Could you check a few things on this model? Use its own coordinates, in mm. Round coordinates to 2 decimals unless told otherwise and drop trailing zeros. Loops run counter-clockwise (first coordinate to the right, second up) from the corner with the lowest first, then second, coordinate; pieces in that order, holes last.
Autodesk Inventor part; units mm, degrees
ref_plane "YZ Plane" through (0, 0, 0) normal (1, 0, 0) x (0, 1, 0)
ref_plane "XZ Plane" through (0, 0, 0) normal (0, 1, 0) x (-1, 0, 0)
ref_plane "XY Plane" through (0, 0, 0) normal (0, 0, 1) x (1, 0, 0)
sketch "Sketch1" plane through (0, 0, 0) normal (0, 1, 0) x (-1, 0, 0)
  line L0 (0, 0) -> (0, -180)
  line L1 (0, -180) -> (-120, -180)
  line L2 (-120, -180) -> (-120, 0)
  line L3 (-120, 0) -> (0, 0)
  dimension "d1" = 180
  dimension "d2" = 120
extrude "Extrusion1" add sketch "Sketch1" along normal blind 1
fillet "Fillet1" radius 2 4 edges at (0, 0.5, 0) (120, 0.5, 0) (120, 0.5, -180) (0, 0.5, -180)
sketch "Sketch2" plane through (0, 1, 0) normal (0, 1, 0) x (1, 0, 0)
  arc A0 (2, 180) -> (0, 178) centre (2, 178) ccw
  circle A1 centre (2.7071, 177.2929) radius 1.5
  line L0 (2, 0) -> (118, 0)
  line L1 (118, 180) -> (2, 180)
  arc A2 (120, 178) -> (118, 180) centre (118, 178) ccw
  circle A3 centre (117.2929, 177.2929) radius 1.5
  arc A4 (118, 0) -> (120, 2) centre (118, 2) ccw
  circle A5 centre (117.2929, 3.7977) radius 1.5
  arc A6 (0, 2) -> (2, 0) centre (2, 2) ccw
  circle A7 centre (2.7071, 2.7071) radius 1.5
  point P0 (0, 0)
  dimension "d7" = 3
  dimension "d10" = 3
  dimension "d11" = 3
extrude "Extrusion2" cut sketch "Sketch2" against normal through all
sketch "Sketch3" plane through (0, 1, 0) normal (0, 1, 0) x (1, 0, 0)
  line L0 (57.2525, 21.6143) -> (70.3337, 21.6143)
  line L1 (70.3337, 21.6143) -> (70.3337, 9.5938)
  line L2 (70.3337, 9.5938) -> (57.2525, 9.5938)
  line L3 (57.2525, 9.5938) -> (57.2525, 21.6143)
  line L4 (84.4572, 173.1647) -> (99.2564, 173.1647)
  line L5 (99.2564, 173.1647) -> (99.2564, 161.3857)
  line L6 (99.2564, 161.3857) -> (84.4572, 161.3857)
  line L7 (84.4572, 161.3857) -> (84.4572, 173.1647)
  point P0 (0, 0)
extrude "Extrusion3" add sketch "Sketch3" along normal blind 10
sketch "Sketch4" plane through (0, 11, 0) normal (0, 1, 0) x (1, 0, 0)
  circle A0 centre (63.7549, 15.2444) radius 2.3335
  circle A1 centre (90.6401, 167.8396) radius 3.0183
  line L0 (57.2525, 9.5938) -> (70.3337, 9.5938)
  line L1 (70.3337, 21.6143) -> (70.3337, 9.5938)
  line L2 (70.3337, 9.5938) -> (57.2525, 9.5938)
  line L3 (57.2525, 9.5938) -> (57.2525, 21.6143)
  line L4 (57.2525, 21.6143) -> (70.3337, 21.6143)
  line L5 (99.2564, 161.3857) -> (99.2564, 173.1647)
  line L6 (84.4572, 173.1647) -> (99.2564, 173.1647)
  line L7 (99.2564, 173.1647) -> (99.2564, 161.3857)
  line L8 (99.2564, 161.3857) -> (84.4572, 161.3857)
  line L9 (84.4572, 173.1647) -> (84.4572, 161.3857)
  line L10 (84.4572, 161.3857) -> (84.4572, 173.1647)
  point P0 (0, 0)
extrude "Extrusion4" cut sketch "Sketch4" against normal blind 7
equation "\"BendRadius\" = Thickness"
equation "\"BendReliefWidth\" = Thickness"
equation "\"BendReliefDepth\" = 0.5 * Thickness"
equation "\"CornerReliefSize\" = 4 * Thickness"
equation "\"MinimumRemnant\" = 2 * Thickness"
equation "\"TransitionRadius\" = BendRadius"
equation "\"JacobiRadiusSize\" = BendRadius"
equation "\"GapSize\" = Thickness"
properties part number "PCB" material "Aluminum 6061"
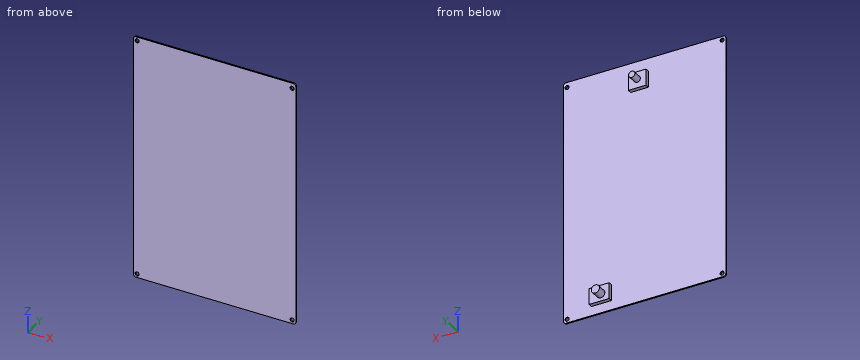
Item 1: If we section it at D-D, the plane z = -49: Please give me the cut outline in (x, y).
Results list:
outline: (0, 0) - (120, 0) - (120, 1) - (0, 1) - close
Item 2: Will these pins go through, and if not, where does the flat tip stop? pin 1 (3.5 mm diameter, centred on x = 61, y = 2, fed in from -Z); pin 2 (3 mm diameter, centred on x = 56, y = 3, fed in from +Z); pin 3 (3.5 mm diameter, centred on x = 2.71, z = -2.71, fed in from +Y); pin 4 (3.5 mm diameter, centred on y = 3, z = -14, fed in from -X).
Results list:
pin 1: stops at z = -180
pin 2: stops at z = -9.59
pin 3: stops at y = 1
pin 4: stops at x = 57.25
Item 3: If we section it at B-B, the plane y = 7.75: Please give me the cut outline in (x, z).
Results list:
outline: circle Ø4.67 at (63.75, -15.24); circle Ø6.04 at (90.64, -167.84)
Item 4: If we section it at A-A, the plane z = -19.5: Please give me the cut outline in (x, y).
Results list:
outline: (0, 0) - (120, 0) - (120, 1) - (70.33, 1) - (70.33, 4) - (57.25, 4) - (57.25, 1) - (0, 1) - close
Item 5: If I drill on line 1 along Y through (x, z) = (31, -124); line 2 along Z through (x, y) = (93, 6.5); line 3 along Z through (x, y) = (89, 8.75), over which ranges is the centre line in solid material (lowest first)?
Results list:
line 1: y = 0 to 1
line 2: z = -169.72 to -165.96
line 3: z = -170.37 to -165.31
Item 6: If we section it at C-C, the plane x = 75: Please give me the cut outline in (y, z).
Results list:
outline: (0, -180) - (1, -180) - (1, 0) - (0, 0) - close
